```python
from build123d import *

# Parameters (mm, degrees)
SKETCH1_W           = 45.72
SKETCH1_H           = 31.75
BOSS_EXTRUDE1_DEPTH = 40.64
SKETCH2_W           = 33.528
SKETCH2_H           = 28.448
CUT_EXTRUDE1_DEPTH  = 3.175
SKETCH3_W           = 6.604
SKETCH3_H           = 6.096
CUT_EXTRUDE2_DEPTH  = 6.604
SKETCH4_W           = 6.604
SKETCH4_H           = 4.445
CUT_EXTRUDE3_DEPTH  = 3.429
SKETCH5_W           = 33.02
SKETCH5_H           = 12.192
CUT_EXTRUDE4_DEPTH  = 50.256520634
SKETCH6_W           = 12.192
SKETCH6_H           = 27.94
CUT_EXTRUDE5_DEPTH  = 64.197655218
FILLET1_R           = 5.08
FILLET2_R           = 5.08
SKETCH7_W           = 45.72
SKETCH7_H           = 31.75
CUT_EXTRUDE6_DEPTH  = 4.572
SKETCH8_W           = 45.72
SKETCH8_H           = 31.75
CUT_EXTRUDE7_DEPTH  = 4.572


with BuildPart() as part:
    # Sketch1 → Boss-Extrude1 (new body)
    with BuildSketch(Plane(origin=(0, 0, 0), x_dir=(1, 0, 0), z_dir=(0, 1, 0))):
        Rectangle(SKETCH1_W, SKETCH1_H)
    extrude(amount=BOSS_EXTRUDE1_DEPTH)

    # Sketch2 → Cut-Extrude1 (cut)
    with BuildSketch(Plane.XY.offset(15.875)):
        with Locations((0, 20.32)):
            Rectangle(SKETCH2_W, SKETCH2_H)
    cut_extrude1 = extrude(amount=-CUT_EXTRUDE1_DEPTH, mode=Mode.SUBTRACT)

    # Sketch3 → Cut-Extrude2 (cut)
    with BuildSketch(Plane.XY.offset(15.875)):
        with Locations((0, 37.592)):
            Rectangle(SKETCH3_W, SKETCH3_H)
        with Locations((0, 3.048)):
            Rectangle(SKETCH3_W, SKETCH3_H)
        with Locations((-12.7, 3.048)):
            Rectangle(SKETCH3_W, SKETCH3_H)
        with Locations((12.7, 3.048)):
            Rectangle(SKETCH3_W, SKETCH3_H)
    cut_extrude2 = extrude(amount=-CUT_EXTRUDE2_DEPTH, mode=Mode.SUBTRACT)

    # Sketch4 → Cut-Extrude3 (cut)
    with BuildSketch(Plane.XY.offset(12.7)):
        with Locations((0, 32.3215)):
            Rectangle(SKETCH4_W, SKETCH4_H)
        with Locations((-12.7, 8.3185)):
            Rectangle(SKETCH4_W, SKETCH4_H)
        with Locations((0, 8.3185)):
            Rectangle(SKETCH4_W, SKETCH4_H)
        with Locations((12.7, 8.3185)):
            Rectangle(SKETCH4_W, SKETCH4_H)
    cut_extrude3 = extrude(amount=-CUT_EXTRUDE3_DEPTH, mode=Mode.SUBTRACT)

    # Mirror1: Cut-Extrude1, Cut-Extrude2, Cut-Extrude3 across plane
    add(cut_extrude1.mirror(Plane.XY), mode=Mode.SUBTRACT)
    add(cut_extrude2.mirror(Plane.XY), mode=Mode.SUBTRACT)
    add(cut_extrude3.mirror(Plane.XY), mode=Mode.SUBTRACT)

    # Sketch5 → Cut-Extrude4 (cut, through all)
    with BuildSketch(Plane(origin=(0, 40.64, 0), x_dir=(1, 0, 0), z_dir=(0, 1, 0))):
        Rectangle(SKETCH5_W, SKETCH5_H)
    extrude(amount=-CUT_EXTRUDE4_DEPTH, mode=Mode.SUBTRACT)

    # Sketch6 → Cut-Extrude5 (cut, through all)
    with BuildSketch(Plane.ZY.offset(22.86)):
        with Locations((0, 20.32)):
            Rectangle(SKETCH6_W, SKETCH6_H)
    extrude(amount=-CUT_EXTRUDE5_DEPTH, mode=Mode.SUBTRACT)

    # Fillet1
    fillet1_edges = [part.edges().sort_by_distance(p)[0] for p in [
        (16.51, 3.175, -6.096),
        (16.51, 3.175, 6.096),
        (-16.51, 3.175, 6.096),
        (-16.51, 3.175, -6.096),
        (-16.51, 37.465, -6.096),
        (16.51, 37.465, -6.096),
        (-16.51, 37.465, 6.096),
        (16.51, 37.465, 6.096),
    ]]
    fillet(fillet1_edges, radius=FILLET1_R)

    # Fillet2
    fillet2_edges = [part.edges().sort_by_distance(p)[0] for p in [
        (-17.145, 6.35, 6.096),
        (-17.145, 6.35, -6.096),
        (-17.145, 34.29, 6.096),
        (-17.145, 34.29, -6.096),
        (17.145, 34.29, 6.096),
        (17.145, 34.29, -6.096),
        (17.145, 6.35, 6.096),
        (17.145, 6.35, -6.096),
    ]]
    fillet(fillet2_edges, radius=FILLET2_R)

    # Sketch7 → Cut-Extrude6 (cut)
    with BuildSketch(Plane(origin=(0, 40.64, 0), x_dir=(1, 0, 0), z_dir=(0, 1, 0))):
        Rectangle(SKETCH7_W, SKETCH7_H)
    extrude(amount=-CUT_EXTRUDE6_DEPTH, mode=Mode.SUBTRACT)

    # Sketch8 → Cut-Extrude7 (cut)
    with BuildSketch(Plane.XZ):
        Rectangle(SKETCH8_W, SKETCH8_H)
    extrude(amount=-CUT_EXTRUDE7_DEPTH, mode=Mode.SUBTRACT)


solid = part.part
```
For this review, take the finished solid that the model builds, in its own axes (mm). A direction names the side the tool comes from. Round coordinates to 2 decimals unless told otherwise and drop trailing zeros. Order: outer loops, then holes, each group sorted by start corner. A loop starts at its lowest first (then second) coordinate and runs counter-clockwise, first axis right, second up.
Q1. We need section B-B, the plane x = -10. Give the boundary of the cut face in (y, z) (3 decimals), plus the area to 3 significant figures.
Findings below:
outline: (4.572, -9.271) - (10.541, -9.271) - (10.541, -12.7) - (34.544, -12.7) - (34.544, -15.875) - (36.068, -15.875) - (36.068, -6.096) - (4.572, -6.096) - close; (4.572, 6.096) - (36.068, 6.096) - (36.068, 15.875) - (34.544, 15.875) - (34.544, 12.7) - (10.541, 12.7) - (10.541, 9.271) - (4.572, 9.271) - close
area: 385 mm2
Q2. Wall thickness on line 1 (X direction, y = 22.5, z = 14.5); line 2 (Z direction, x = 10, y = 20); line 3 (Z direction, x = -19, y = 24) (3 decimals): over which ranges is each line inside the solid? List them lowest first.
Findings below:
line 1: x = -22.86 to -16.76, 16.76 to 22.86
line 2: z = -12.7 to -6.1, 6.1 to 12.7
line 3: z = -15.875 to -6.096, 6.096 to 15.875
Q3. Machinability: for faces 4 (the cylindrical face through (-14.3, 34.11, -5.21)), 5 (the flat face through (-20, 6.35, 0)), 6 (the flat face through (13, 10.541, -11)), 7 (the flat face through (3.302, 34, 12)), 8 (the flat face through (-6, 6.096, -14)), which of the approach directions +Z, -Z, +X, -X, +Y, -Y give a long, thin tool a straight path to every point of the face, cutting with its end or side? Answer none if there is none.
Findings below:
face 4: +Y, -Y
face 5: +X, -X
face 6: -Z, -Y
face 7: +Z, +Y
face 8: -Z
Q4. We need section D-D, the plane x = -20. Give the boundary of the cut face in (y, z) (3 decimals).
Findings below:
outline: (4.572, -15.875) - (36.068, -15.875) - (36.068, 15.875) - (4.572, 15.875) - close; hole (6.35, -1.016) arc R5.08 ccw to (11.43, -6.096) - (29.21, -6.096) arc R5.08 ccw to (34.29, -1.016) - (34.29, 1.016) arc R5.08 ccw to (29.21, 6.096) - (11.43, 6.096) arc R5.08 ccw to (6.35, 1.016) - close
Q5. Insertion check: P1, Ø3, axis at x = 9.5, y = 28, coming from the +Z side; P2, Ø1, axis at x = 0.5, z = 11.5, coming from the +Y side; P3, Ø2.5, axis at x = -0.5, z = 11, coming from the -Y side. Each pin has a flat end and moves straight along its axis. Give the tip position at first contact, or say it passes through.
Findings below:
P1: stops at z = 12.7
P2: stops at y = 30.1
P3: stops at y = 10.54
Q6. Mouldability with a two-part tool opening along Z and no side actions: class faces 1 (the flat face through (-3.302, 34, -12)), 2 (the cylindrical face through (14.3, 6.43, -5.21)), 3 (the flat face through (-6, 5, 15.875)) as pulls with the +Z half, pulls with the -Z half, needs draft (parallel to the pull), parting line crosses it, or undercut.
Findings below:
face 1: needs draft
face 2: undercut
face 3: pulls with the +Z half
Q7. We need section A-A, the plane y = 20. Give the boundary of the cut face in (x, z) (3 decimals).
Findings below:
outline: (-22.86, -15.875) - (-16.764, -15.875) - (-16.764, -12.7) - (16.764, -12.7) - (16.764, -15.875) - (22.86, -15.875) - (22.86, -6.096) - (-22.86, -6.096) - close; (-22.86, 6.096) - (22.86, 6.096) - (22.86, 15.875) - (16.764, 15.875) - (16.764, 12.7) - (-16.764, 12.7) - (-16.764, 15.875) - (-22.86, 15.875) - close
Q8. We need section C-C, the plane z = -5.5. Give the boundary of the cut face in (x, y).
Findings below:
outline: (-22.86, 4.57) - (-13.82, 4.57) - (-13.82, 9.04) - (-22.86, 9.04) - close; (-22.86, 31.6) - (-13.82, 31.6) - (-13.82, 36.07) - (-22.86, 36.07) - close; (13.82, 4.57) - (22.86, 4.57) - (22.86, 9.04) - (13.82, 9.04) - close; (13.82, 31.6) - (22.86, 31.6) - (22.86, 36.07) - (13.82, 36.07) - close
